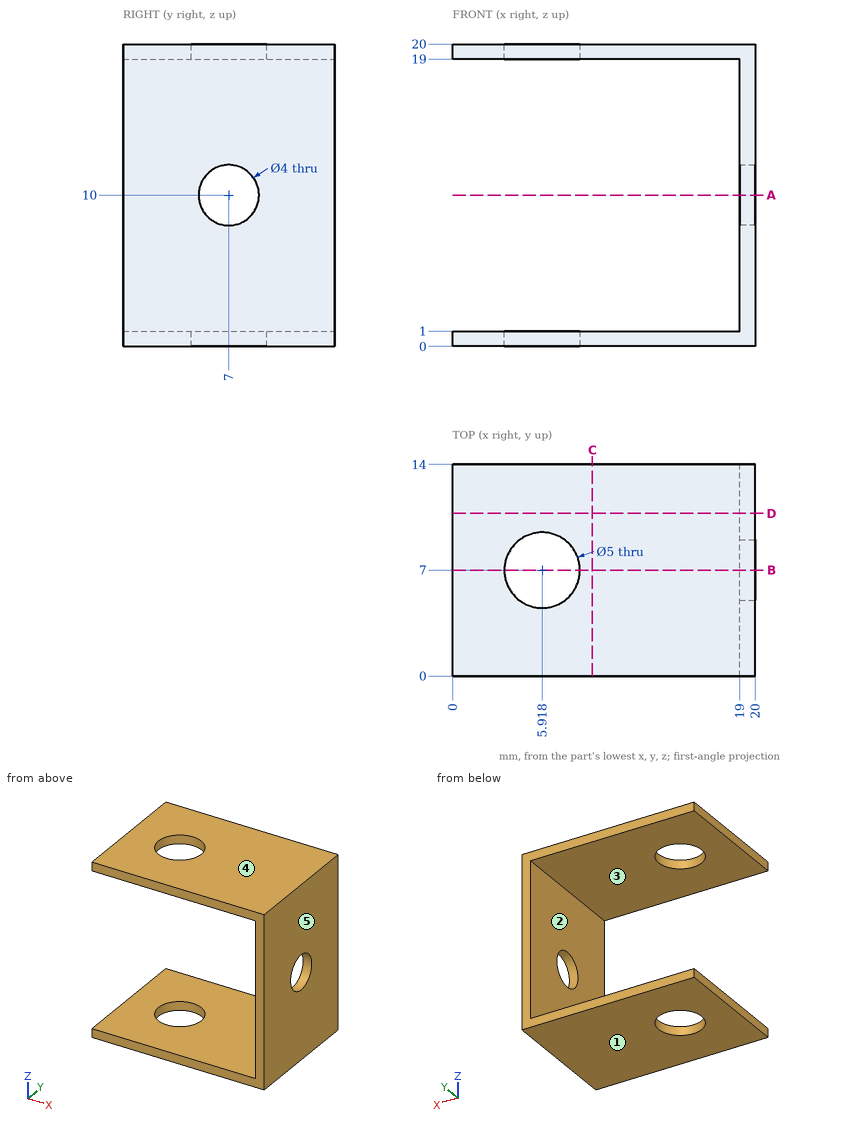
Job drawing, mm, ordinate dimensions from the low corner. One solid piece. A direction names the side the tool comes from. Coordinates: 2 decimals unless noted, no trailing zeros. Loops run counter-clockwise (first coordinate to the right, second up) from the corner with the lowest first, then second, coordinate; pieces in that order, holes last. Notation, with made-up numbers: (-10, -16) - (19, -16) arc R10 ccw to (19, -3) - close; hole circle Ø11 at (28, 35.25). An arc over 180 degrees is marked (long way). Answer as a JSON object with one key per item and string values. Group by question number.
(1) Cut at B-B (y = 7). Give the cut face in (x, z).
(2) Cut at A-A (z = 10). Give the cut face in (x, y), then the cut area to 3 significant figures.
(3) Two-plate mould, pull along Z, no slides. Class the marked faces 3, 4 and 5: released by +Z, released by -Z, zero draft, split by the parting line, or undercut.
(4) Flat gauge pins, fed straight in: pin 1 (4 mm diameter, centred on y = 6.5, z = 5.5, fed in from -X); pin 2 (4 mm diameter, centred on x = 5.92, y = 7, fed in from -Z). Where does each tip first touch, or does it go through?
(5) Cut at D-D (y = 10.75). Give the cut face in (x, z).
(6) Cut at C-C (x = 9.25). Give the cut face in (y, z), then the cut area to 3 significant figures.
(7) Tool access for the marked faces 1 and 2: list every direction of +Z, -Z, +X, -X, +Y, -Y with a clear straight run to the whole face (end or side of a thin tool).
(8) Probe line 1 along Z through (x, y) = (7.5, 10.75); line 2 along Y through (x, z) = (19.35, 10); line 3 along X through (y, z) = (8.5, 6.25). List the from-to ranges inside material, lowest first.
Geometry says:
{
 "1": {"outline": "(0, 0) - (3.42, 0) - (3.42, 1) - (0, 1) - close; (0, 19) - (3.42, 19) - (3.42, 20) - (0, 20) - close; (8.42, 0) - (20, 0) - (20, 8) - (19, 8) - (19, 1) - (8.42, 1) - close; (8.42, 19) - (19, 19) - (19, 12) - (20, 12) - (20, 20) - (8.42, 20) - close"},
 "2": {"outline": "(19, 0) - (20, 0) - (20, 5) - (19, 5) - close; (19, 9) - (20, 9) - (20, 14) - (19, 14) - close", "area": "10.0 mm^2"},
 "3": {"face 3": "undercut", "face 4": "released by +Z", "face 5": "zero draft"},
 "4": {"pin 1": "stops at x = 19", "pin 2": "passes through"},
 "5": {"outline": "(0, 0) - (20, 0) - (20, 20) - (0, 20) - (0, 19) - (19, 19) - (19, 1) - (0, 1) - close"},
 "6": {"outline": "(0, 0) - (14, 0) - (14, 1) - (0, 1) - close; (0, 19) - (14, 19) - (14, 20) - (0, 20) - close", "area": "28.0 mm^2"},
 "7": {"face 1": "-Z, +X, -X, +Y, -Y", "face 2": "-X, +Y, -Y"},
 "8": {"line 1": "z = 0 to 1, 19 to 20", "line 2": "y = 0 to 5, 9 to 14", "line 3": "x = 19 to 20"}
}
